```python
from build123d import *

# Parameters (mm, degrees)
BOSS_EXTRUDE1_DEPTH     = 15
CUT_EXTRUDE1_DEPTH      = 61.415229868
CUT_EXTRUDE1_DEPTH_BACK = 61.415229868
SKETCH2_R               = 12.5
FILLET2_R               = 5
FILLET3_R               = 20


with BuildPart() as part:
    # Sketch1 → Boss-Extrude1 (new body)
    with BuildSketch(Plane(origin=(0, 0, 0), x_dir=(1, 0, 0), z_dir=(0, 1, 0))):
        Polygon((-10, 20), (15, 10), (15, -10), (-10, -20), (-55, -20), (-55, 20), align=None)
    extrude(amount=BOSS_EXTRUDE1_DEPTH)

    # Sketch2 → Cut-Extrude1 (cut, two sides: drawn at the far end of the back side and taken through both)
    with BuildSketch(Plane.XY.offset(-CUT_EXTRUDE1_DEPTH_BACK)):
        with Locations((-30.5, 0)):
            Circle(SKETCH2_R)
    extrude(amount=CUT_EXTRUDE1_DEPTH + CUT_EXTRUDE1_DEPTH_BACK, mode=Mode.SUBTRACT)

    # Fillet2
    fillet2_edges = [part.edges().sort_by_distance(p)[0] for p in [
        (-55, 7.5, 20),
        (-55, 7.5, -20),
        (15, 7.5, -10),
        (15, 7.5, 10),
    ]]
    fillet(fillet2_edges, radius=FILLET2_R)

    # Fillet3
    fillet3_edges = [part.edges().sort_by_distance(p)[0] for p in [
        (-10, 7.5, 20),
        (-10, 7.5, -20),
    ]]
    fillet(fillet3_edges, radius=FILLET3_R)


solid = part.part
```
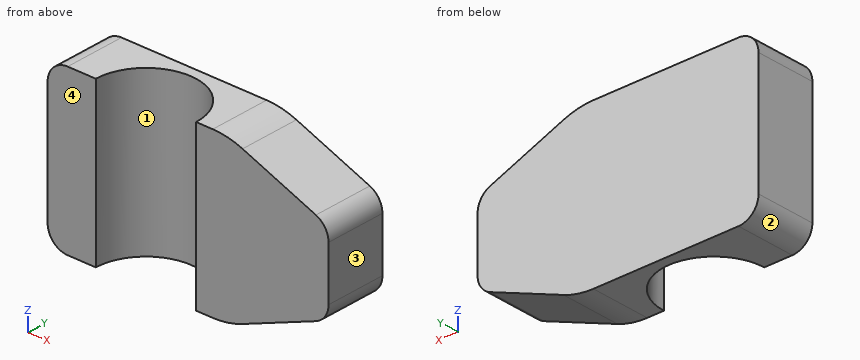
Verification items for the finished model (mm, model axes). Face numbers are marked on the shaded views. Round coordinates to 2 decimals unless told otherwise and drop trailing zeros. Write each loop counter-clockwise with the first axis right and the second up, starting at its lowest first coordinate (ties: lowest second). Pieces come first, ordered by that corner, then holes.
1. Section check A-A on y = 9. Enter the section's corners in (x, z), plus the area to 3 significant figures.
2. Section check D-D on y = 6. Enter the section's corners in (x, z), plus the area to 3 significant figures.
3. Scan lines: L1, parallel to X at y = 8, z = 10.5; L2, parallel to X at y = 3.75, z = -4.5; L3, parallel to Y at x = -30, z = -7.5. Record each from-to range of solid material in increasing order.
4. Draft check along X on the marked faces 1, 2, 3 and 4. Enter one of: +X half, -X half, draft (parallel to the pull), parting line (faces both ways), or undercut.
5. Gauge pin test, flat ends, axial feed: P1, Ø3, axis at y = 5, z = 9.5, coming from the +X side; P2, Ø10, axis at x = -33, z = 15.5, coming from the -Y side. Record the tip position at first contact, or that the pin passes through.
6. Section check B-B on z = 3. Enter the section's corners in (x, y).
7. Section check C-C on x = -30.5. Enter the section's corners in (y, z).
Answer:
1. outline: (-55, -15) arc R5 ccw to (-50, -20) - (-39.17, -20) - (-39.17, 20) - (-50, 20) arc R5 ccw to (-55, 15) - close; (-21.83, -20) - (-13.85, -20) arc R20 ccw to (-6.42, -18.57) - (11.86, -11.26) arc R5 ccw to (15, -6.61) - (15, 6.61) arc R5 ccw to (11.86, 11.26) - (-6.42, 18.57) arc R20 ccw to (-13.85, 20) - (-21.83, 20) - close
1. area: 1,840 mm2
2. outline: (-55, -15) arc R5 ccw to (-50, -20) - (-41.47, -20) - (-41.47, 20) - (-50, 20) arc R5 ccw to (-55, 15) - close; (-19.53, -20) - (-13.85, -20) arc R20 ccw to (-6.42, -18.57) - (11.86, -11.26) arc R5 ccw to (15, -6.61) - (15, 6.61) arc R5 ccw to (11.86, 11.26) - (-6.42, 18.57) arc R20 ccw to (-13.85, 20) - (-19.53, 20) - close
2. area: 1,660 mm2
3. L1: x = -55 to -40.1, -20.9 to 13.15
3. L2: x = -55 to -42.42, -18.58 to 15
3. L3: y = 12.49 to 15
4. face 1: undercut
4. face 2: -X half
4. face 3: +X half
4. face 4: draft
5. P1: stops at x = 14.8
5. P2: stops at y = 10
6. outline: (-55, 0) - (-43, 0) arc R12.5 cw to (-18, 0) - (15, 0) - (15, 15) - (-55, 15) - close
7. outline: (12.5, -20) - (15, -20) - (15, 20) - (12.5, 20) - close
